from build123d import *

# Parameters (mm, degrees)
ESQUISSE1_R             = 10.75
ESQUISSE1_R_2           = 3.675
BOSS_EXTRU_1_DEPTH      = 60
ESQUISSE2_W             = 50
ESQUISSE2_H             = 29
ENL_V_MAT_EXTRU_1_DEPTH = 58.75
D_GAGEMENT_M21_D        = 2.6
ESQUISSE4_R             = 6.35
ENL_V_MAT_EXTRU_2_DEPTH = 4
ENL_V_START             = -4
ESQUISSE5_R             = 6.35
ENL_V_MAT_EXTRU_3_DEPTH = 4


with BuildPart() as part:
    # Esquisse1 → Boss.-Extru.1 (new body)
    with BuildSketch(Plane(origin=(0, 0, 0), x_dir=(1, 0, 0), z_dir=(0, 1, 0))):
        with BuildLine():
            Line((-53.54472285, -18), (-53.54472285, -41.100032298))
            ThreePointArc((-53.54472285, -41.100032298), (67.5, 0), (-53.54472285, 41.100032298))
            Line((-53.54472285, 41.100032298), (-53.54472285, 18))
            Line((-53.54472285, 18), (-98.54472285, 18))
            ThreePointArc((-98.54472285, 18), (-107.66, 0), (-98.54472285, -18))
            Line((-98.54472285, -18), (-53.54472285, -18))
        make_face()
        with Locations(Location((-85.33, 0, 0), (0, 0, 270))):
            Circle(ESQUISSE1_R, mode=Mode.SUBTRACT)
        with Locations(Location((0, 0, 0), (0, 0, 270))):
            Circle(ESQUISSE1_R_2, mode=Mode.SUBTRACT)
    extrude(amount=BOSS_EXTRU_1_DEPTH)

    # Esquisse2 → Enlèv. mat.-Extru.1 (cut)
    with BuildSketch(Plane.XZ):
        with Locations((-71.58, 0)):
            Rectangle(ESQUISSE2_W, ESQUISSE2_H)
    extrude(amount=-ENL_V_MAT_EXTRU_1_DEPTH, mode=Mode.SUBTRACT)

    # Dégagement M21 (through all)
    with Locations(Plane(origin=(-56.83, 47.5, -18), x_dir=(-1, 0, 0), z_dir=(0, 0, -1))):
        with Locations((0, 0), (24, 0), (24, -12), (0, -12)):
            Hole(D_GAGEMENT_M21_D / 2)

    # Esquisse4 → Enlèv. mat.-Extru.2 (cut)
    with BuildSketch(Plane.XZ):
        with Locations(Location((0, 0, 0), (0, 0, 270))):
            Circle(ESQUISSE4_R)
    extrude(amount=-ENL_V_MAT_EXTRU_2_DEPTH, mode=Mode.SUBTRACT)

    # Esquisse5 → Enlèv. mat.-Extru.3 (cut)
    with BuildSketch(Plane(origin=(0, 60, 0), x_dir=(1, 0, 0), z_dir=(0, 1, 0)).offset(ENL_V_START)):
        with Locations(Location((0, 0, 0), (0, 0, 90))):
            Circle(ESQUISSE5_R)
    extrude(amount=ENL_V_MAT_EXTRU_3_DEPTH, mode=Mode.SUBTRACT)


solid = part.part
Verification items for the finished model (mm, model axes). A direction names the side the tool comes from. Coordinates: 2 decimals unless noted, no trailing zeros. Write each loop counter-clockwise with the first axis right and the second up, starting at its lowest first coordinate (ties: lowest second). Pieces come first, ordered by that corner, then holes. Notation, with made-up numbers: M 6.25,62.25 L 35.25,62.25 A31 ccw 35.25,90.25 Z; hole C 61,47.5 d7. An arc over 180 degrees is marked long. Use a Markdown table: item, result.
Q1. Sectioned sample at A-A, the plane x = 0. Record the boundary of the cut face in (y, z) (3 decimals), plus the area to 3 significant figures.
Reply:
| item | result |
|---|---|
| outline | M 0,-67.5 L 60,-67.5 L 60,-6.35 L 56,-6.35 L 56,-3.675 L 4,-3.675 L 4,-6.35 L 0,-6.35 Z; M 0,6.35 L 4,6.35 L 4,3.675 L 56,3.675 L 56,6.35 L 60,6.35 L 60,67.5 L 0,67.5 Z |
| area | 7,620 mm² |
Q2. Go/stop test with flat-tipped pins: P1, Ø14.5, axis at y = 20.5, z = 7, coming from the -X side; P2, Ø12, axis at y = 24, z = -29, coming from the -X side; P3, Ø12, axis at x = -1, y = 17, coming from the -Z side. Record where each tip stops, or that it passes through.
Reply:
| item | result |
|---|---|
| P1 | stops at x = -107.66 |
| P2 | stops at x = -53.54 |
| P3 | stops at z = -67.5 |
Q3. Draft check along Z on faces 5 (the face through (-21, 60, -1)), 6 (the face through (-72, 29, 14.5)), 7 (the face through (-76, 30, -18)). Enter one of: +Z half, -Z half, draft (parallel to the pull), parting line (faces both ways), or undercut.
Reply:
| item | result |
|---|---|
| face 5 | draft |
| face 6 | undercut |
| face 7 | -Z half |
Q4. Thickness scan on line 1 (Y direction, x = -56.83, z = -16.1); line 2 (X direction, y = 56.95, z = 0); line 3 (X direction, y = 58.8, z = 0). Record the ranges inside material, lowest first.
Reply:
| item | result |
|---|---|
| line 1 | y = 0 to 34.2, 36.8 to 46.2, 48.8 to 60 |
| line 2 | x = -107.66 to -96.58, -46.58 to -6.35, 6.35 to 67.5 |
| line 3 | x = -107.66 to -96.08, -74.58 to -6.35, 6.35 to 67.5 |
Q5. Sectioned sample at C-C, the plane x = -66. Record the boundary of the cut face in (y, z), plus the area to 3 significant figures.
Reply:
| item | result |
|---|---|
| outline | M 0,-18 L 60,-18 L 60,18 L 0,18 L 0,14.5 L 58.75,14.5 L 58.75,-14.5 L 0,-14.5 Z |
| area | 456 mm² |
Q6. Set-up check for faces 1 (the face through (-53.545, 30, 29)), 2 (the face through (-96.58, 29, 0)), 3 (the face through (-53.545, 30, -30)), 4 (the face through (3, 56, -3)): record each of +Z, -Z, +X, -X, +Y, -Y from which the full face is reachable in a straight line by a thin tool's end or side.
Reply:
| item | result |
|---|---|
| face 1 | +Z, -X, +Y, -Y |
| face 2 | -Y |
| face 3 | -Z, -X, +Y, -Y |
| face 4 | +Y |
Q7. Sectioned sample at D-D, the plane x = -92. Record the boundary of the cut face in (y, z), plus the area to 3 significant figures.
Reply:
| item | result |
|---|---|
| outline | M 0,-18 L 60,-18 L 60,-8.43 L 58.75,-8.43 L 58.75,-14.5 L 0,-14.5 Z; M 0,14.5 L 58.75,14.5 L 58.75,8.43 L 60,8.43 L 60,18 L 0,18 Z |
| area | 435 mm² |
Q8. Sectioned sample at B-B, the plane y = 31.5. Record the boundary of the cut face in (x, z) (3 decimals).
Reply:
| item | result |
|---|---|
| outline | M -98.545,-18 L -53.545,-18 L -53.545,-41.1 A67.5 ccw long -53.545,41.1 L -53.545,18 L -98.545,18 A22.33 ccw Z; hole M -96.58,-14.5 L -46.58,-14.5 L -46.58,14.5 L -96.58,14.5 Z; hole C 0,0 d7.35 |
